Here's the drawing with two shaded views (mm, measured from the low corner). I have some questions. A direction names the side the tool comes from. Give positions to 0.01 mm unless a question says otherwise; leave off trailing zeros. Write each loop counter-clockwise with the first axis right and the second up, starting at its lowest first coordinate (ties: lowest second). Pieces come first, ordered by that corner, then holes. Notation, with made-up numbers: (45.25, -5) - (94.25, -5) arc R15 ccw to (94.25, 15) - close; hole circle Ø1 at (48.5, 44). An arc over 180 degrees is marked (long way). Answer as a JSON object with one key per item and string values. Group by question number.
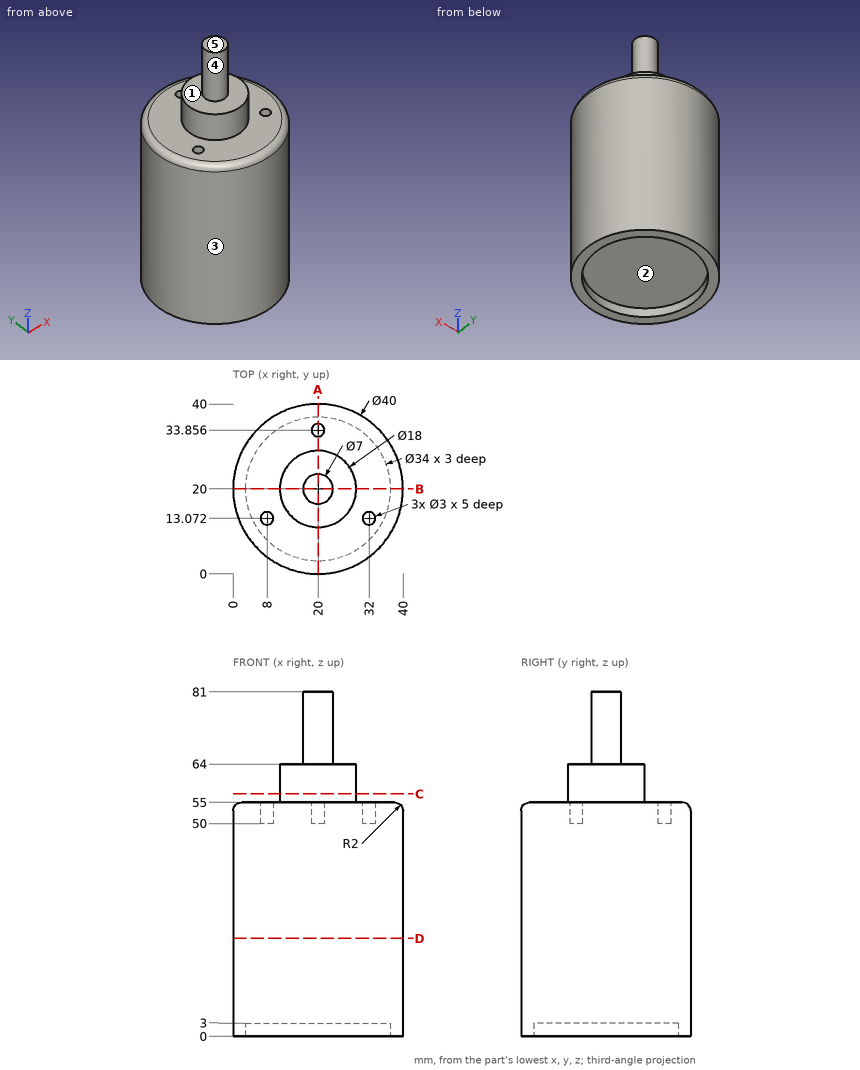
(1) I want a section at A-A, the plane x = 20. Please give me the cut outline in (y, z), and give its area (3 significant figures).
(2) I want a section at C-C, the plane z = 57. Please give me the cut outline in (x, y).
(3) I want a section at D-D, the plane z = 23. Please give me the cut outline in (x, y).
(4) Will these pins go through, and if not, where does the flat tip stop? P1, Ø1.5, axis at x = 15, z = 19.5, coming from the -Y side; P2, Ø3.5, axis at x = 19.5, y = 34.5, coming from the +Z side; P3, Ø1.5, axis at x = 8.5, y = 13, coming from the +Z side.
(5) I need wall thicknesses on L1, parallel to Y at x = 20, z = 1.2; L2, parallel to Y at x = 20, z = 51.45; L3, parallel to Z at x = 10, y = 22. Which ranges of each line are inside material? Lowest first, please.
(6) I want a section at B-B, the plane y = 20. Please give me the cut outline in (x, z).
(7) For the marked faces 4 and 5, which set-ups out of +Z, -Z, +X, -X, +Y, -Y let a thin tool reach every point of the face, with its end or its side?
(8) If we mould it in two halves opening along Y, with no side actions, what happens to the marked faces 1, 2 and 3? For each: +Y half, -Y half, draft (parallel to the pull), parting line (faces both ways), or undercut.
Entries:
{
 "1": {"outline": "(0, 0) - (3, 0) - (3, 3) - (37, 3) - (37, 0) - (40, 0) - (40, 53) arc R2 ccw to (38, 55) - (35.36, 55) - (35.36, 50) - (32.36, 50) - (32.36, 55) - (29, 55) - (29, 64) - (23.5, 64) - (23.5, 81) - (16.5, 81) - (16.5, 64) - (11, 64) - (11, 55) - (2, 55) arc R2 ccw to (0, 53) - close", "area": "2,360 mm^2"},
 "2": {"outline": "circle Ø18 at (20, 20)"},
 "3": {"outline": "circle Ø40 at (20, 20)"},
 "4": {"P1": "y = 0.46", "P2": "z = 55", "P3": "z = 50"},
 "5": {"L1": "0 to 3, 37 to 40", "L2": "0 to 32.36, 35.36 to 40", "L3": "3 to 55"},
 "6": {"outline": "(0, 0) - (3, 0) - (3, 3) - (37, 3) - (37, 0) - (40, 0) - (40, 53) arc R2 ccw to (38, 55) - (29, 55) - (29, 64) - (23.5, 64) - (23.5, 81) - (16.5, 81) - (16.5, 64) - (11, 64) - (11, 55) - (2, 55) arc R2 ccw to (0, 53) - close"},
 "7": {"face 4": "+Z", "face 5": "+Z, +X, -X, +Y, -Y"},
 "8": {"face 1": "draft", "face 2": "undercut", "face 3": "parting line"}
}
